```python
from build123d import *

# Parameters (mm, degrees)
BOSS_EXTRUDE1_DEPTH = 5
SKETCH3_W           = 40
SKETCH3_H           = 10
BOSS_EXTRUDE2_DEPTH = 5
SKETCH4_W           = 40
SKETCH4_H           = 5
BOSS_EXTRUDE3_DEPTH = 4
SKETCH7_W           = 10
SKETCH7_H           = 6.2
CUT_EXTRUDE1_DEPTH  = 75.540257579
SKETCH8_R           = 2
CUT_EXTRUDE2_DEPTH  = 6
FILLET3_R           = 5


with BuildPart() as part:
    # Sketch1 → Boss-Extrude1 (new, symmetric)
    with BuildSketch(Plane.XY):
        Polygon((5, -57.5), (30, -57.5), (30, -67.5), (-30, -67.5), (-30, -57.5), (-5, -57.5), (-5, 57.5), (-20, 57.5), (-20, 62.5), (20, 62.5), (20, 57.5), (5, 57.5), align=None)
    extrude(amount=BOSS_EXTRUDE1_DEPTH, both=True)

    # Sketch3 → Boss-Extrude2 (add)
    with BuildSketch(Plane(origin=(0, 62.5, 0), x_dir=(1, 0, 0), z_dir=(0, 1, 0))):
        with Locations((0, -10)):
            Rectangle(SKETCH3_W, SKETCH3_H)
    extrude(amount=-BOSS_EXTRUDE2_DEPTH)

    # Sketch4 → Boss-Extrude3 (add)
    with BuildSketch(Plane(origin=(0, 62.5, 0), x_dir=(1, 0, 0), z_dir=(0, 1, 0))):
        with Locations((0, -12.5)):
            Rectangle(SKETCH4_W, SKETCH4_H)
    extrude(amount=BOSS_EXTRUDE3_DEPTH)

    # Sketch7 → Cut-Extrude1 (cut, through all)
    with BuildSketch(Plane.XY.offset(5)):
        with Locations((0, -64.4)):
            Rectangle(SKETCH7_W, SKETCH7_H)
    extrude(amount=-CUT_EXTRUDE1_DEPTH, mode=Mode.SUBTRACT)

    # Sketch8 → Cut-Extrude2 (cut)
    with BuildSketch(Plane.XZ.offset(61.3)):
        with Locations(Location((0, 0, 0), (0, 0, 270))):
            Circle(SKETCH8_R)
    extrude(amount=-CUT_EXTRUDE2_DEPTH, mode=Mode.SUBTRACT)

    # Fillet3
    fillet3_edges = [part.edges().sort_by_distance(p)[0] for p in [
        (5, -57.5, 0),
        (-5, -57.5, 0),
        (-5, 57.5, 0),
        (5, 57.5, 0),
        (0, 57.5, 5),
    ]]
    fillet(fillet3_edges, radius=FILLET3_R)


solid = part.part
```
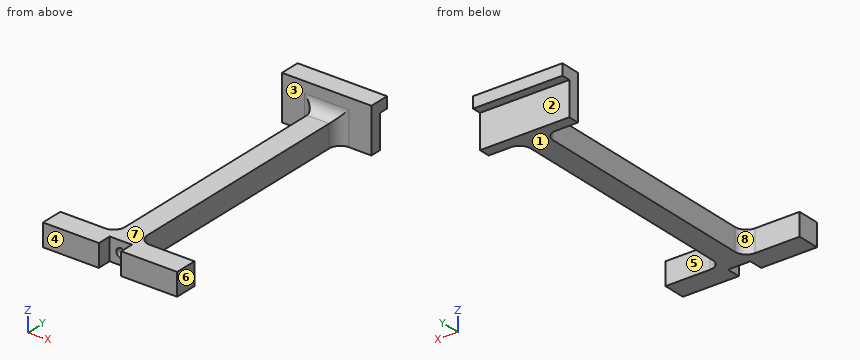
Can you work these out from the model? Positions are in its coordinate system, mm. Face numbers are marked on the shaded views. A direction names the side the tool comes from. Round coordinates to 2 decimals unless told otherwise and drop trailing zeros. Loops run counter-clockwise (first coordinate to the right, second up) from the corner with the lowest first, then second, coordinate; pieces in that order, holes last. Notation, with made-up numbers: M 52.5,-3 L 79.5,-3 A16 cw 79.5,16 Z; hole C 73.25,30 d9. An arc over 180 degrees is marked long. Answer as a JSON object with one key per item and string values. Group by question number.
Q1. We'd pull the mould along Y, two halves only. Please class the marked faces 1, 2 and 3: +Y half, -Y half, draft (parallel to the pull), parting line (faces both ways), or undercut.
Q2. Imagine slicing it at A-A, the plane x = 15.5. Please give me the cut outline in (y, z), then the cut area to 3 significant figures.
Q3. On a 3-axis mill with a long thin cutter (end or side, diameter ignored), from which of +Z, -Z, +X, -X, +Y, -Y can I reach the whole of each face in a straight line? I mean the marked faces 4, 5, 6, 7 and 8. Say none if no direction works.
Q4. Will these pins go through, and if not, where does the flat tip stop? pin 1 (7 mm diameter, centred on y = 64, z = 4.5, fed in from -X); pin 2 (12 mm diameter, centred on y = 16, z = -1.5, fed in from -X); pin 3 (2.5 mm diameter, centred on y = 61.5, z = 9.5, fed in from +X); pin 4 (11 mm diameter, centred on x = -1.5, z = 0, fed in from -Y).
Q5. Imagine slicing it at D-D, the plane y = 6. Please give me the cut outline in (x, z), then the cut area to 3 significant figures.
Q6. Please list where these lines run through material, in increasing order: L1, parallel to X at y = -58.35, z = 0; L2, parallel to Y at x = -17, z = 8.25; L3, parallel to X at y = 11, z = -1.75.
Q7. Imagine slicing it at B-B, the plane x = 0. Please give me the cut outline in (y, z).
Q8. Imagine slicing it at C-C, the plane z = 0. Please give me the cut outline in (x, y).
Findings:
{
 "1": {"face 1": "draft", "face 2": "+Y half", "face 3": "undercut"},
 "2": {"outline": "M -67.5,-5 L -57.5,-5 L -57.5,5 L -67.5,5 Z; M 57.5,-5 L 62.5,-5 L 62.5,10 L 66.5,10 L 66.5,15 L 57.5,15 Z", "area": "220 mm2"},
 "3": {"face 4": "+Z, -Z, +X, -X, -Y", "face 5": "+Z, -Z, +X", "face 6": "+Z, -Z, +X, +Y, -Y", "face 7": "+Z, +X, -X, -Y", "face 8": "+Z, -Z, -X"},
 "4": {"pin 1": "stops at x = -20", "pin 2": "stops at x = -5", "pin 3": "stops at x = 20", "pin 4": "stops at y = -67.5"},
 "5": {"outline": "M -5,-5 L 5,-5 L 5,5 L -5,5 Z", "area": "100 mm2"},
 "6": {"L1": "x = -30 to -2, 2 to 30", "L2": "y = 57.5 to 62.5", "L3": "x = -5 to 5"},
 "7": {"outline": "M -61.3,-5 L 62.5,-5 L 62.5,10 L 66.5,10 L 66.5,15 L 57.5,15 L 57.5,10 A5 cw 52.5,5 L -61.3,5 L -61.3,2 L -55.3,2 L -55.3,-2 L -61.3,-2 Z"},
 "8": {"outline": "M -30,-67.5 L -5,-67.5 L -5,-61.3 L -2,-61.3 L -2,-55.3 L 2,-55.3 L 2,-61.3 L 5,-61.3 L 5,-67.5 L 30,-67.5 L 30,-57.5 L 10,-57.5 A5 cw 5,-52.5 L 5,52.5 A5 cw 10,57.5 L 20,57.5 L 20,62.5 L -20,62.5 L -20,57.5 L -10,57.5 A5 cw -5,52.5 L -5,-52.5 A5 cw -10,-57.5 L -30,-57.5 Z"}
}
